from build123d import *

# Parameters (mm, degrees)
SKETCH1_W          = 25.4
SKETCH1_H          = 25.4
BASE_EXTRUDE_DEPTH = 298.45
FILLET1_R          = 3.175
SHELL1_T           = -1.5875
SKETCH4_R          = 3.175
CUT_EXTRUDE1_DEPTH = 26.4
CUT_EXTRUDE3_REACH = 3.588
SKETCH6_R          = 2.5


with BuildPart() as part:
    # Sketch1 → Base-Extrude (new body, symmetric)
    with BuildSketch(Plane.XY):
        Rectangle(SKETCH1_W, SKETCH1_H)
    extrude(amount=BASE_EXTRUDE_DEPTH, both=True)

    # Fillet1
    fillet1_edges = [part.edges().sort_by_distance(p)[0] for p in [
        (-12.7, 12.7, 0),
        (12.7, 12.7, 0),
        (12.7, -12.7, 0),
        (-12.7, -12.7, 0),
    ]]
    fillet(fillet1_edges, radius=FILLET1_R)

    # Shell1
    shell1_openings = [part.faces().sort_by_distance(p)[0] for p in [
        (0, 0, 298.45),
        (0, 0, -298.45),
    ]]
    offset(amount=SHELL1_T, openings=shell1_openings, kind=Kind.INTERSECTION)

    # Sketch4 → Cut-Extrude1 (cut, through all)
    with BuildSketch(Plane.XZ.offset(12.7)):
        with Locations((0, 273.05)):
            Circle(SKETCH4_R)
        with Locations((0, 247.65)):
            Circle(SKETCH4_R)
        with Locations((0, -247.65)):
            Circle(SKETCH4_R)
        with Locations((0, -273.05)):
            Circle(SKETCH4_R)
    extrude(amount=-CUT_EXTRUDE1_DEPTH, mode=Mode.SUBTRACT)

    # Sketch6 → Cut-Extrude3 (cut, up to next)
    with BuildSketch(Plane.ZY.offset(-11.1125), mode=Mode.PRIVATE) as cut_extrude3_sk1:
        with Locations((-95.25, 0)):
            Circle(SKETCH6_R)
    cut_extrude3_tool1 = extrude(cut_extrude3_sk1.sketch, amount=-CUT_EXTRUDE3_REACH, mode=Mode.PRIVATE) & part.part
    add(cut_extrude3_tool1.solids().sort_by_distance((11.1125, 0, -95.25))[0], mode=Mode.SUBTRACT)
    # Sketch6 → Cut-Extrude3 (cut, up to next)
    with BuildSketch(Plane.ZY.offset(-11.1125), mode=Mode.PRIVATE) as cut_extrude3_sk2:
        with Locations((-222.25, 0)):
            Circle(SKETCH6_R)
    cut_extrude3_tool2 = extrude(cut_extrude3_sk2.sketch, amount=-CUT_EXTRUDE3_REACH, mode=Mode.PRIVATE) & part.part
    add(cut_extrude3_tool2.solids().sort_by_distance((11.1125, 0, -222.25))[0], mode=Mode.SUBTRACT)
    # Sketch6 → Cut-Extrude3 (cut, up to next)
    with BuildSketch(Plane.ZY.offset(-11.1125), mode=Mode.PRIVATE) as cut_extrude3_sk3:
        with Locations((222.25, 0)):
            Circle(SKETCH6_R)
    cut_extrude3_tool3 = extrude(cut_extrude3_sk3.sketch, amount=-CUT_EXTRUDE3_REACH, mode=Mode.PRIVATE) & part.part
    add(cut_extrude3_tool3.solids().sort_by_distance((11.1125, 0, 222.25))[0], mode=Mode.SUBTRACT)
    # Sketch6 → Cut-Extrude3 (cut, up to next)
    with BuildSketch(Plane.ZY.offset(-11.1125), mode=Mode.PRIVATE) as cut_extrude3_sk4:
        with Locations((95.25, 0)):
            Circle(SKETCH6_R)
    cut_extrude3_tool4 = extrude(cut_extrude3_sk4.sketch, amount=-CUT_EXTRUDE3_REACH, mode=Mode.PRIVATE) & part.part
    add(cut_extrude3_tool4.solids().sort_by_distance((11.1125, 0, 95.25))[0], mode=Mode.SUBTRACT)


solid = part.part
Source: CAD feature listing. Evaluate the final solid. Frame: model axes, mm. A direction names the side the tool comes from. Give positions to 0.01 mm unless a question says otherwise; leave off trailing zeros. Return JSON: item names as keys, results as strings. Group by question number.
1) Set-up query: faces 5 (the face through (-11.112, 0, 4)), 6 (the face through (-11.3, 1, -298.45)). Return all of +Z, -Z, +X, -X, +Y, -Y with unobstructed straight access to the full face (end or side cutting, diameter ignored); none if empty.
2) Material intervals for line 1 along Z through (x, y) = (0, 11.7) (3 decimals); line 2 along X through (y, z) = (8.5, -45), sorted ascending. Write a range as [from, to].
3) Pull-direction query (X, two-part tool) for faces 1 (the face through (12.7, 0, 4)), 2 (the face through (11.112, 0, 4)), 3 (the face through (-12.7, 0, 4)), 4 (the face through (-11.3, 1, 298.45)); classes: pulls with the +X half, pulls with the -X half, needs draft (parallel to the pull), parting line crosses it, or undercut.
Recorded:
{
 "1": {"face 5": "+Z, -Z", "face 6": "-Z, +X, -X, +Y, -Y"},
 "2": {"line 1": "z = [-298.45, -276.225], [-269.875, -250.825], [-244.475, 244.475], [250.825, 269.875], [276.225, 298.45]", "line 2": "x = [-12.7, -11.11], [11.11, 12.7]"},
 "3": {"face 1": "pulls with the +X half", "face 2": "undercut", "face 3": "pulls with the -X half", "face 4": "needs draft"}
}
